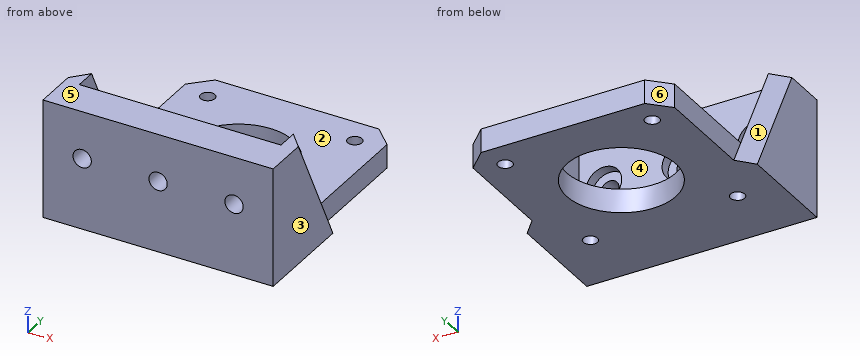
from build123d import *

# Parameters (mm, degrees)
SKETCH1_W           = 42.5
SKETCH1_H           = 42.5
SKETCH1_R           = 1.5
SKETCH1_R_2         = 11.5
BOSS_EXTRUDE1_DEPTH = 5
CHAMFER1_SIZE       = 4
SKETCH2_W           = 42.5
SKETCH2_H           = 25
BOSS_EXTRUDE2_DEPTH = 8
BOSS_EXTRUDE3_DEPTH = 3
SKETCH4_R           = 3.75
CUT_EXTRUDE1_DEPTH  = 2.2
SKETCH5_R           = 1.925
CUT_EXTRUDE2_DEPTH  = 57.667031862


with BuildPart() as part:
    # Sketch1 → Boss-Extrude1 (new body)
    with BuildSketch(Plane.XY):
        Rectangle(SKETCH1_W, SKETCH1_H)
        with Locations((15.5, 15.5)):
            Circle(SKETCH1_R, mode=Mode.SUBTRACT)
        with Locations(Location((-15.5, 15.5, 0), (0, 0, 180))):
            Circle(SKETCH1_R, mode=Mode.SUBTRACT)
        with Locations(Location((15.5, -15.5, 0), (0, 0, 180))):
            Circle(SKETCH1_R, mode=Mode.SUBTRACT)
        with Locations((-15.5, -15.5)):
            Circle(SKETCH1_R, mode=Mode.SUBTRACT)
        Circle(SKETCH1_R_2, mode=Mode.SUBTRACT)
    extrude(amount=BOSS_EXTRUDE1_DEPTH)

    # Chamfer1
    chamfer1_edges = [part.edges().sort_by_distance(p)[0] for p in [
        (-21.25, 21.25, 2.5),
        (21.25, 21.25, 2.5),
    ]]
    chamfer(chamfer1_edges, length=CHAMFER1_SIZE)

    # Sketch2 → Boss-Extrude2 (add)
    with BuildSketch(Plane.XZ.offset(21.25)):
        with Locations((0, 12.5)):
            Rectangle(SKETCH2_W, SKETCH2_H)
    extrude(amount=BOSS_EXTRUDE2_DEPTH)

    # Sketch3 → Boss-Extrude3 (add)
    with BuildSketch(Plane(origin=(21.25, 0, 0), x_dir=(0, 0, -1), z_dir=(1, 0, 0))):
        Polygon((-25, -21.25), (0, -8.681713823), (0, -29.25), (-25, -29.25), align=None)
    boss_extrude3 = extrude(amount=BOSS_EXTRUDE3_DEPTH)

    # Mirror3: Boss-Extrude3 across plane
    add(boss_extrude3.mirror(Plane(origin=(0, 0, 0), x_dir=(0, 0, 1), z_dir=(1, 0, 0))))

    # Chamfer2
    # the kernel refuses this chamfer: 4 mm, written as the material it adds along each edge
    with BuildSketch(Plane(origin=(-21.25, -22.284423421, 27.057606356), x_dir=(-0.9996219169112968, -0.02456616062709099, -0.012350181481602638), z_dir=(0, 0.44916485684431295, -0.8934488969023511))) as chamfer2_piece_1_section:
        with BuildLine():
            Line((4.114692781, 0), (-0.22618862, 4.108471174))
            Line((-0.22618862, 4.108471174), (-0.306158373, 4.106271504))
            ThreePointArc((-0.306158373, 4.106271504), (-0.136516908, 2.053591319), (-0.079969753, -0.00219967))
            Line((-0.079969753, -0.00219967), (0.00219967, -0.079969753))
            ThreePointArc((0.00219967, -0.079969753), (2.057990659, -0.023422598), (4.116892451, -0.079969753))
            Line((4.116892451, -0.079969753), (4.114692781, 0))
        make_face()
    chamfer2_piece_1 = extrude(amount=54.972604346, mode=Mode.PRIVATE)
    chamfer2_piece_1 = split(chamfer2_piece_1, bisect_by=Plane(origin=(-24.25, -14.705039529, 15), z_dir=(1, 0, 0)), keep=Keep.TOP, mode=Mode.PRIVATE)
    chamfer2_piece_1 = split(chamfer2_piece_1, bisect_by=Plane(origin=(-22.462839724, -14.705039529, 25), z_dir=(0, 0, -1)), keep=Keep.TOP, mode=Mode.PRIVATE)
    chamfer2_piece_1 = split(chamfer2_piece_1, bisect_by=Plane(origin=(-21.25, -14.705039529, 15), z_dir=(-1, 0, 0)), keep=Keep.TOP, mode=Mode.PRIVATE)
    chamfer2_piece_1 = split(chamfer2_piece_1, bisect_by=Plane(origin=(-22.462839724, -14.705039529, 5), z_dir=(0, 0, 1)), keep=Keep.TOP, mode=Mode.PRIVATE)
    add(chamfer2_piece_1)
    with BuildSketch(Plane(origin=(-21.25, -22.284423421, 27.057606356), x_dir=(-0.9996219169112968, -0.02456616062709099, -0.012350181481602638), z_dir=(0, 0.44916485684431295, -0.8934488969023511))) as chamfer2_piece_2_section:
        with BuildLine():
            Line((4.114692781, 0), (-0.22618862, 4.108471174))
            Line((-0.22618862, 4.108471174), (-0.306158373, 4.106271504))
            ThreePointArc((-0.306158373, 4.106271504), (-0.136516908, 2.053591319), (-0.079969753, -0.00219967))
            Line((-0.079969753, -0.00219967), (0.00219967, -0.079969753))
            ThreePointArc((0.00219967, -0.079969753), (2.057990659, -0.023422598), (4.116892451, -0.079969753))
            Line((4.116892451, -0.079969753), (4.114692781, 0))
        make_face()
    chamfer2_piece_2 = extrude(amount=54.972604346, mode=Mode.PRIVATE)
    chamfer2_piece_2 = split(chamfer2_piece_2, bisect_by=Plane(origin=(-24.25, -8.42089644, 2.5), z_dir=(1, 0, 0)), keep=Keep.TOP, mode=Mode.PRIVATE)
    chamfer2_piece_2 = split(chamfer2_piece_2, bisect_by=Plane(origin=(-22.462839724, -8.42089644, 0), z_dir=(0, 0, 1)), keep=Keep.TOP, mode=Mode.PRIVATE)
    chamfer2_piece_2 = split(chamfer2_piece_2, bisect_by=Plane(origin=(-21.25, -8.42089644, 2.5), z_dir=(-1, 0, 0)), keep=Keep.TOP, mode=Mode.PRIVATE)
    chamfer2_piece_2 = split(chamfer2_piece_2, bisect_by=Plane(origin=(-22.462839724, -8.42089644, 5), z_dir=(0, 0, -1)), keep=Keep.TOP, mode=Mode.PRIVATE)
    add(chamfer2_piece_2)
    with BuildSketch(Plane(origin=(-21.25, -22.284423421, 27.057606356), x_dir=(-0.9996219169112968, -0.02456616062709099, -0.012350181481602638), z_dir=(0, 0.44916485684431295, -0.8934488969023511))) as chamfer2_piece_3_section:
        with BuildLine():
            Line((4.114692781, 0), (-0.22618862, 4.108471174))
            Line((-0.22618862, 4.108471174), (-0.306158373, 4.106271504))
            ThreePointArc((-0.306158373, 4.106271504), (-0.136516908, 2.053591319), (-0.079969753, -0.00219967))
            Line((-0.079969753, -0.00219967), (0.00219967, -0.079969753))
            ThreePointArc((0.00219967, -0.079969753), (2.057990659, -0.023422598), (4.116892451, -0.079969753))
            Line((4.116892451, -0.079969753), (4.114692781, 0))
        make_face()
    chamfer2_piece_3 = extrude(amount=54.972604346, mode=Mode.PRIVATE)
    chamfer2_piece_3 = split(chamfer2_piece_3, bisect_by=Plane(origin=(-21.193688037, -7.24875826, 0), z_dir=(0, 0, 1)), keep=Keep.TOP, mode=Mode.PRIVATE)
    chamfer2_piece_3 = split(chamfer2_piece_3, bisect_by=Plane(origin=(-21.25, -7.24875826, 2.5), z_dir=(1, 0, 0)), keep=Keep.TOP, mode=Mode.PRIVATE)
    chamfer2_piece_3 = split(chamfer2_piece_3, bisect_by=Plane(origin=(-21.193688037, -7.24875826, 5), z_dir=(0, 0, -1)), keep=Keep.TOP, mode=Mode.PRIVATE)
    add(chamfer2_piece_3)
    with BuildSketch(Plane(origin=(21.25, -22.284423421, 27.057606356), x_dir=(-0.027495876610586504, 0.8931110989838116, 0.4489950352079003), z_dir=(0, 0.44916485684431295, -0.8934488969023511))) as chamfer2_piece_4_section:
        with BuildLine():
            Line((4.114692781, 0), (-0.22618862, 4.108471174))
            Line((-0.22618862, 4.108471174), (-0.306158373, 4.106271504))
            ThreePointArc((-0.306158373, 4.106271504), (-0.136516908, 2.053591319), (-0.079969753, -0.00219967))
            Line((-0.079969753, -0.00219967), (0.00219967, -0.079969753))
            ThreePointArc((0.00219967, -0.079969753), (2.057990659, -0.023422598), (4.116892451, -0.079969753))
            Line((4.116892451, -0.079969753), (4.114692781, 0))
        make_face()
    chamfer2_piece_4 = extrude(amount=54.972604346, mode=Mode.PRIVATE)
    chamfer2_piece_4 = split(chamfer2_piece_4, bisect_by=Plane(origin=(22.462839724, -14.705039529, 5), z_dir=(0, 0, 1)), keep=Keep.TOP, mode=Mode.PRIVATE)
    chamfer2_piece_4 = split(chamfer2_piece_4, bisect_by=Plane(origin=(22.462839724, -14.705039529, 25), z_dir=(0, 0, -1)), keep=Keep.TOP, mode=Mode.PRIVATE)
    chamfer2_piece_4 = split(chamfer2_piece_4, bisect_by=Plane(origin=(21.25, -14.705039529, 15), z_dir=(1, 0, 0)), keep=Keep.TOP, mode=Mode.PRIVATE)
    chamfer2_piece_4 = split(chamfer2_piece_4, bisect_by=Plane(origin=(24.25, -14.705039529, 15), z_dir=(-1, 0, 0)), keep=Keep.TOP, mode=Mode.PRIVATE)
    add(chamfer2_piece_4)
    with BuildSketch(Plane(origin=(21.25, -22.284423421, 27.057606356), x_dir=(-0.027495876610586504, 0.8931110989838116, 0.4489950352079003), z_dir=(0, 0.44916485684431295, -0.8934488969023511))) as chamfer2_piece_5_section:
        with BuildLine():
            Line((4.114692781, 0), (-0.22618862, 4.108471174))
            Line((-0.22618862, 4.108471174), (-0.306158373, 4.106271504))
            ThreePointArc((-0.306158373, 4.106271504), (-0.136516908, 2.053591319), (-0.079969753, -0.00219967))
            Line((-0.079969753, -0.00219967), (0.00219967, -0.079969753))
            ThreePointArc((0.00219967, -0.079969753), (2.057990659, -0.023422598), (4.116892451, -0.079969753))
            Line((4.116892451, -0.079969753), (4.114692781, 0))
        make_face()
    chamfer2_piece_5 = extrude(amount=54.972604346, mode=Mode.PRIVATE)
    chamfer2_piece_5 = split(chamfer2_piece_5, bisect_by=Plane(origin=(21.193688037, -7.24875826, 0), z_dir=(0, 0, 1)), keep=Keep.TOP, mode=Mode.PRIVATE)
    chamfer2_piece_5 = split(chamfer2_piece_5, bisect_by=Plane(origin=(21.193688037, -7.24875826, 5), z_dir=(0, 0, -1)), keep=Keep.TOP, mode=Mode.PRIVATE)
    chamfer2_piece_5 = split(chamfer2_piece_5, bisect_by=Plane(origin=(21.25, -7.24875826, 2.5), z_dir=(-1, 0, 0)), keep=Keep.TOP, mode=Mode.PRIVATE)
    add(chamfer2_piece_5)
    with BuildSketch(Plane(origin=(21.25, -22.284423421, 27.057606356), x_dir=(-0.027495876610586504, 0.8931110989838116, 0.4489950352079003), z_dir=(0, 0.44916485684431295, -0.8934488969023511))) as chamfer2_piece_6_section:
        with BuildLine():
            Line((4.114692781, 0), (-0.22618862, 4.108471174))
            Line((-0.22618862, 4.108471174), (-0.306158373, 4.106271504))
            ThreePointArc((-0.306158373, 4.106271504), (-0.136516908, 2.053591319), (-0.079969753, -0.00219967))
            Line((-0.079969753, -0.00219967), (0.00219967, -0.079969753))
            ThreePointArc((0.00219967, -0.079969753), (2.057990659, -0.023422598), (4.116892451, -0.079969753))
            Line((4.116892451, -0.079969753), (4.114692781, 0))
        make_face()
    chamfer2_piece_6 = extrude(amount=54.972604346, mode=Mode.PRIVATE)
    chamfer2_piece_6 = split(chamfer2_piece_6, bisect_by=Plane(origin=(22.462839724, -8.42089644, 0), z_dir=(0, 0, 1)), keep=Keep.TOP, mode=Mode.PRIVATE)
    chamfer2_piece_6 = split(chamfer2_piece_6, bisect_by=Plane(origin=(22.462839724, -8.42089644, 5), z_dir=(0, 0, -1)), keep=Keep.TOP, mode=Mode.PRIVATE)
    chamfer2_piece_6 = split(chamfer2_piece_6, bisect_by=Plane(origin=(21.25, -8.42089644, 2.5), z_dir=(1, 0, 0)), keep=Keep.TOP, mode=Mode.PRIVATE)
    chamfer2_piece_6 = split(chamfer2_piece_6, bisect_by=Plane(origin=(24.25, -8.42089644, 2.5), z_dir=(-1, 0, 0)), keep=Keep.TOP, mode=Mode.PRIVATE)
    add(chamfer2_piece_6)

    # Sketch4 → Cut-Extrude1 (cut)
    with BuildSketch(Plane(origin=(0, -21.25, 0), x_dir=(1, 0, 0), z_dir=(0, 1, 0))):
        with Locations(Location((0, -15, 0), (0, 0, 270))):
            Circle(SKETCH4_R)
        with Locations(Location((16, -15, 0), (0, 0, 270))):
            Circle(SKETCH4_R)
        with Locations(Location((-16, -15, 0), (0, 0, 270))):
            Circle(SKETCH4_R)
    extrude(amount=-CUT_EXTRUDE1_DEPTH, mode=Mode.SUBTRACT)

    # Sketch5 → Cut-Extrude2 (cut, through all)
    with BuildSketch(Plane(origin=(0, -23.45, 0), x_dir=(1, 0, 0), z_dir=(0, 1, 0))):
        with Locations(Location((0, -15, 0), (0, 0, 270))):
            Circle(SKETCH5_R)
        with Locations(Location((16, -15, 0), (0, 0, 270))):
            Circle(SKETCH5_R)
        with Locations(Location((-16, -15, 0), (0, 0, 270))):
            Circle(SKETCH5_R)
    extrude(amount=-CUT_EXTRUDE2_DEPTH, mode=Mode.SUBTRACT)


solid = part.part
Work out the finished part from the listing and answer in its coordinate system (mm). Face numbers are marked on the shaded views. A direction names the side the tool comes from. Round coordinates to 2 decimals unless told otherwise and drop trailing zeros. Order: outer loops, then holes, each group sorted by start corner. A loop starts at its lowest first (then second) coordinate and runs counter-clockwise, first axis right, second up. Notation, with made-up numbers: M -18.5,3.25 L 33.5,3.25 A20 cw 33.5,17.25 Z; hole C -0.5,35 d10. An arc over 180 degrees is marked long. One line per item, written item: value.
Q1. Straight lines are drawn through the part: line 1 (X direction, y = -22.5, z = 15); line 2 (Y direction, x = -15.5, z = 1.45); line 3 (X direction, y = -27.25, z = 15) (3 decimals). For each, find the intervals that lie inside material, in ascending order.
Derived:
line 1: -24.25 to -19.75, -12.25 to -3.75, 3.75 to 12.25, 19.75 to 24.25
line 2: -29.25 to -17, -14 to 14, 17 to 21.25
line 3: -24.25 to -17.925, -14.075 to -1.925, 1.925 to 14.075, 17.925 to 24.25
Q2. Find section B-B on x = 16. Write down the section's boundary in (y, z) (3 decimals).
Derived:
outline: M -29.25,0 L -16.914,0 L -16.914,5 L -21.25,5 L -21.25,11.25 L -23.45,11.25 L -23.45,13.075 L -29.25,13.075 Z; M -29.25,16.925 L -23.45,16.925 L -23.45,18.75 L -21.25,18.75 L -21.25,25 L -29.25,25 Z; M -14.086,0 L 14.086,0 L 14.086,5 L -14.086,5 Z; M 16.914,0 L 21.25,0 L 21.25,5 L 16.914,5 Z
Q3. For the marked faces 1 and 2, determine the directions among +Z, -Z, +X, -X, +Y, -Y from which every point of the face is accessible in a straight line to the end or side of a thin tool.
Derived:
face 1: +Z, -X, +Y
face 2: +Z, +Y
Q4. Find section D-D on x = 3. Write down the section's boundary in (y, z).
Derived:
outline: M -29.25,0 L -11.1,0 L -11.1,5 L -21.25,5 L -21.25,12.75 L -23.45,12.75 L -23.45,17.25 L -21.25,17.25 L -21.25,25 L -29.25,25 Z; M 11.1,0 L 21.25,0 L 21.25,5 L 11.1,5 Z
Q5. Find section A-A on y = 0. Write down the section's boundary in (x, z), then the cut area to 3 significant figures.
Derived:
outline: M -21.25,0 L -11.5,0 L -11.5,5 L -21.25,5 Z; M 11.5,0 L 21.25,0 L 21.25,5 L 11.5,5 Z
area: 97.5 mm²
Q6. Find section C-C on y = -15.5. Write down the section's boundary in (x, z).
Derived:
outline: M -24.25,0 L -17,0 L -17,5 L -21.25,5 L -21.25,22.47 L -24.25,15.79 Z; M -14,0 L 14,0 L 14,5 L -14,5 Z; M 17,0 L 24.25,0 L 24.25,15.79 L 21.25,22.47 L 21.25,5 L 17,5 Z
Q7. Flat-ended cylindrical pins translate along their axes: pin 1 (1.5 mm diameter, centred on y = 4, z = 2.5, fed in from -X); pin 2 (7 mm diameter, centred on x = 16, z = 15, fed in from +Y); pin 3 (5 mm diameter, centred on x = -15.5, y = -15.5, fed in from +Z). Find the tip coordinate at first contact, or state that the pin passes through.
Derived:
pin 1: x = -21.25
pin 2: y = -23.45
pin 3: z = 5
Q8. Determine the mould class of the marked faces 3, 4, 5 and 6 for opening direction X: released by +X, released by -X, zero draft, split by the parting line, or undercut.
Derived:
face 3: released by +X
face 4: undercut
face 5: zero draft
face 6: released by -X
